from build123d import *

# Parameters (mm, degrees)
BOSS_EXTRUDE1_DEPTH                     = 45
BOSS_EXTRUDE2_DEPTH                     = 19
BOSS_EXTRUDE3_DEPTH                     = 10
FILLET1_R                               = 19
CBORE_FOR_M5_HEX_HEAD_BOLT1_D           = 10
CBORE_FOR_M5_HEX_HEAD_BOLT1_DEPTH       = 20
CBORE_FOR_M5_HEX_HEAD_BOLT1_CBORE_D     = 20
CBORE_FOR_M5_HEX_HEAD_BOLT1_CBORE_DEPTH = 6
CBORE_FOR_M5_HEX_HEAD_BOLT1_TIP         = 2.886751346


with BuildPart() as part:
    # Sketch1 → Boss-Extrude1 (new body)
    with BuildSketch(Plane.XY):
        Polygon((100, 13), (0, 13), (0, 0), (63, 0), (63, -6), (100, -6), align=None)
    extrude(amount=BOSS_EXTRUDE1_DEPTH)

    # Sketch1_3 → Boss-Extrude2 (add)
    with BuildSketch(Plane.XY):
        with BuildLine():
            Line((0, 51), (0, 13))
            Line((0, 13), (38, 13))
            Line((38, 13), (38, 51))
            ThreePointArc((38, 51), (36.032775759, 59.419296285), (30.538468428, 66.095156386))
            ThreePointArc((30.538468428, 66.095156386), (10.580703715, 68.032775759), (0, 51))
        make_face()
        with BuildLine():
            Line((9.5, 32), (9.5, 51))
            ThreePointArc((9.5, 51), (19, 60.5), (28.5, 51))
            Line((28.5, 51), (28.5, 32))
            ThreePointArc((28.5, 32), (19, 22.5), (9.5, 32))
        make_face(mode=Mode.SUBTRACT)
    extrude(amount=BOSS_EXTRUDE2_DEPTH)

    # Sketch1_4 → Boss-Extrude3 (add)
    with BuildSketch(Plane.XY):
        with BuildLine():
            Line((38, 51), (38, 13))
            Line((38, 13), (100, 13))
            Line((100, 13), (30.538468428, 66.095156386))
            ThreePointArc((30.538468428, 66.095156386), (36.032775759, 59.419296285), (38, 51))
        make_face()
    extrude(amount=BOSS_EXTRUDE3_DEPTH)

    # Fillet1
    fillet1_edges = [part.edges().sort_by_distance(p)[0] for p in [
        (100, 3.5, 45),
    ]]
    fillet(fillet1_edges, radius=FILLET1_R)

    # CBORE for M5 Hex Head Bolt1
    with Locations(Plane(origin=(0, 13, 0), x_dir=(1, 0, 0), z_dir=(0, 1, 0))):
        with Locations((81, -26)):
            CounterBoreHole(CBORE_FOR_M5_HEX_HEAD_BOLT1_D / 2, CBORE_FOR_M5_HEX_HEAD_BOLT1_CBORE_D / 2, CBORE_FOR_M5_HEX_HEAD_BOLT1_CBORE_DEPTH, depth=CBORE_FOR_M5_HEX_HEAD_BOLT1_DEPTH)
            with Locations((0, 0, -(CBORE_FOR_M5_HEX_HEAD_BOLT1_DEPTH + CBORE_FOR_M5_HEX_HEAD_BOLT1_TIP / 2))):  # 120° drill point
                Cone(0, CBORE_FOR_M5_HEX_HEAD_BOLT1_D / 2, CBORE_FOR_M5_HEX_HEAD_BOLT1_TIP, mode=Mode.SUBTRACT)


solid = part.part
Geometry: final body of the model. Coordinates: model frame, mm. A direction names the side the tool comes from. Give positions to 0.01 mm unless a question says otherwise; leave off trailing zeros. Loops run counter-clockwise (first coordinate to the right, second up) from the corner with the lowest first, then second, coordinate; pieces in that order, holes last. Notation, with made-up numbers: M 63,-4 L 86,-4 A21 cw 86,20 Z; hole C -19.75,-4 d2. An arc over 180 degrees is marked long. Put each result on its own line as item: value.
1) Material intervals for L1, parallel to Z at x = 81, y = -2; L2, parallel to Z at x = 81, y = 8.6; L3, parallel to Y at x = 18.5, z = 14, sorted ascending. Write a range as from..to.
Computed values:
L1: z = 0..21, 31..45
L2: z = 0..16, 36..45
L3: y = 0..22.51, 60.49..69.99
2) Cut plane C-C, the plane z = 29. Return the cut outline in (x, y), plus the area to 3 significant figures.
Computed values:
outline: M 0,0 L 63,0 L 63,-6 L 77,-6 L 77,7 L 71.46,7 L 71.46,13 L 0,13 Z; M 85,-6 L 99.76,-6 L 99.76,13 L 90.54,13 L 90.54,7 L 85,7 Z
area: 1,300 mm^2
3) First-contact query: P1, Ø11.5, axis at x = 81, z = 26, coming from the +Y side; P2, Ø19, axis at x = 17, y = 34, coming from the +Z side; P3, Ø7, axis at y = 29, z = 15, coming from the +X side. Flat tips, straight axial feed; report the tip coordinate or a pass-through.
Computed values:
P1: stops at y = 7
P2: stops at z = 19
P3: stops at x = 38
4) Cut plane B-B, the plane y = 47.5. Return the cut outline in (x, z).
Computed values:
outline: M 0,0 L 9.5,0 L 9.5,19 L 0,19 Z; M 28.5,0 L 54.87,0 L 54.87,10 L 38,10 L 38,19 L 28.5,19 Z
5) Reachability of faces 5 (the flat face through (63, -3, 22)), 6 (the flat face through (77, -6, 22)), 7 (the cylindrical face through (18.791, 60.498, 9.367)), 8 (the flat face through (57, 28, 10)) from +Z, -Z, +X, -X, +Y, -Y: full face, straight path, thin tool, end or side. Return the list, or none.
Computed values:
face 5: +Z, -Z, -X, -Y
face 6: +Z, -Z, +X, -X, -Y
face 7: +Z, -Z
face 8: +Z, +X, +Y
6) Cut plane A-A, the plane x = 19. Return the cut outline in (y, z).
Computed values:
outline: M 0,0 L 22.5,0 L 22.5,19 L 13,19 L 13,45 L 0,45 Z; M 60.5,0 L 70,0 L 70,19 L 60.5,19 Z
7) Cut plane D-D, the plane y = 8.5. Return the cut outline in (x, z).
Computed values:
outline: M 0,0 L 100,0 L 100,26 A19 ccw 81,45 L 0,45 Z; hole C 81,26 d20
8) Mould query, pull axis Z, two halves, no side actions, for faces 1 (the cylindrical face through (19.209, 22.502, 9.367)), 2 (the cylindrical face through (76.381, 0.409, 27.915)), 3 (the flat face through (6, 42, 19)), 4 (the cylindrical face through (71, 10, 26)). Classes: released by +Z, released by -Z, zero draft, split by the parting line, or undercut.
Computed values:
face 1: zero draft
face 2: undercut
face 3: released by +Z
face 4: undercut
